Check sheet for the modelled part. Datum: model origin and axes. Units: mm. Face numbers are marked on the shaded views. A direction names the side the tool comes from. Coordinates: 2 decimals unless noted, no trailing zeros. Loops run counter-clockwise (first coordinate to the right, second up) from the corner with the lowest first, then second, coordinate; pieces in that order, holes last. Notation, with made-up numbers: (-14, 45.25) -> (12, 45.25) arc R28 cw to (12, 70.25) -> close; hole circle Ø3 at (85, -10). An arc over 180 degrees is marked (long way). Use one line per item in the form item = value.
from build123d import *

# Parameters (mm, degrees)
F0_W      = 38.7000013143
F0_H      = 33.3000021055
F1_DEPTH  = 25
F3_DEPTH  = 33.3010021055
F4_R      = 50
F5_R      = 0.5
F6_W      = 27.6561714709
F6_H      = 20.6264536828
F7_DEPTH  = 4
F8_W      = 27.6561714709
F8_H      = 16.4114236832
F9_DEPTH  = 10
F10_W     = 27.6561714709
F10_H     = 13.9069892466
F11_DEPTH = 6
F12_W     = 1.1095879599
F12_H     = 33.3000021055
F13_DEPTH = 5


with BuildPart() as f1:
    # F0 (on Top) → F1 (new body)
    with BuildSketch(Plane.XY):
        with Locations((4.9499990419, -5.3999996744)):
            Rectangle(F0_W, F0_H)
    extrude(amount=F1_DEPTH)

    # F2 (on face) → F3 (cut, through all)
    with BuildSketch(Plane.XZ.offset(22.0500007272)):
        Polygon((-14.4000016153, 25), (-14.4000016153, 0), (-3.1048920937, 13.0713665858), (18.2830113918, 19.4805841893), (24.299999699, 25), align=None)
    extrude(amount=-F3_DEPTH, mode=Mode.SUBTRACT)

    # F4
    f4_edges = [f1.edges().sort_by_distance(p)[0] for p in [
        (-3.104892, -5.4, 13.071367),
    ]]
    fillet(f4_edges, radius=F4_R)

    # F5
    f5_edges = [f1.edges().sort_by_distance(p)[0] for p in [
        (24.3, -5.4, 25),
    ]]
    fillet(f5_edges, radius=F5_R)

    # F6 (on face) → F7 (cut)
    with BuildSketch(Plane.YZ.offset(24.299999699)):
        with Locations((-5.37536107, 10.3132268414)):
            Rectangle(F6_W, F6_H)
    extrude(amount=-F7_DEPTH, mode=Mode.SUBTRACT)

    # F8 (on face) → F9 (cut)
    with BuildSketch(Plane.YZ.offset(20.299999699)):
        with Locations((-5.37536107, 8.2057118416)):
            Rectangle(F8_W, F8_H)
    extrude(amount=-F9_DEPTH, mode=Mode.SUBTRACT)

    # F10 (on face) → F11 (cut)
    with BuildSketch(Plane.YZ.offset(10.299999699)):
        with Locations((-5.37536107, 6.9534946233)):
            Rectangle(F10_W, F10_H)
    extrude(amount=-F11_DEPTH, mode=Mode.SUBTRACT)

    # F12 (on face) → F13 (join)
    with BuildSketch(Plane(origin=(0, 0, 0), x_dir=(1, 0, 0), z_dir=(0, 0, -1))):
        with Locations((-13.8452076353, 5.3999996744)):
            Rectangle(F12_W, F12_H)
    extrude(amount=F13_DEPTH)


solid = f1.part
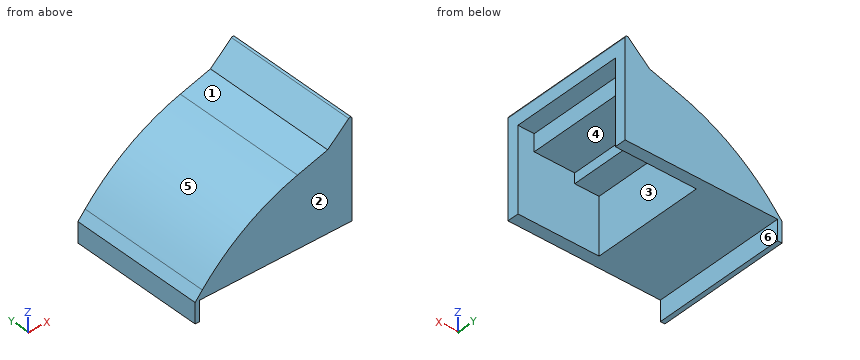
(1) Scan lines: line 1 along Y through (x, z) = (6, 6); line 2 along X through (y, z) = (-18.5, -1.5); line 3 along Z through (x, y) = (2, 8). Record each from-to range of solid material in increasing order.
Established:
line_1 = -22.05 to -19.2, 8.45 to 11.25
line_2 = -14.4 to -13.29
line_3 = 0 to 13.65
(2) Tool access check on the marked faces 4, 5 and 6. Record the directions out of +Z, -Z, +X, -X, +Y, -Y that give a thin tool (end or side, any length) a straight path to the whole face; none if there is none.
Established:
face_4 = -Z, +X
face_5 = +Z, -X, +Y, -Y
face_6 = -Z, +X, +Y, -Y
(3) Section check A-A, the plane y = 0.5. Record the boundary of the cut face in (x, z), plus the area to 3 significant figures.
Established:
outline = (-14.4, -5) -> (-13.29, -5) -> (-13.29, 0) -> (4.3, 0) -> (4.3, 13.91) -> (10.3, 13.91) -> (10.3, 16.41) -> (20.3, 16.41) -> (20.3, 20.63) -> (24.3, 20.63) -> (24.3, 23.86) arc R0.5 ccw to (23.46, 24.23) -> (18.28, 19.48) -> (10.85, 17.25) arc R50 ccw to (-12.63, 2.05) -> (-14.4, 0) -> close
area = 211 mm²
(4) Section check C-C, the plane z = 9.25. Record the boundary of the cut face in (x, y), plus the area to 3 significant figures.
Established:
outline = (-4.94, -22.05) -> (24.3, -22.05) -> (24.3, -19.2) -> (4.3, -19.2) -> (4.3, 8.45) -> (24.3, 8.45) -> (24.3, 11.25) -> (-4.94, 11.25) -> close
area = 421 mm²
(5) Section check D-D, the plane z = -0.5. Record the boundary of the cut face in (x, y).
Established:
outline = (-14.4, -22.05) -> (-13.29, -22.05) -> (-13.29, 11.25) -> (-14.4, 11.25) -> close
(6) Section check B-B, the plane x = 13. Record the boundary of the cut face in (y, z).
Established:
outline = (-22.05, 0) -> (-19.2, 0) -> (-19.2, 16.41) -> (8.45, 16.41) -> (8.45, 0) -> (11.25, 0) -> (11.25, 17.9) -> (-22.05, 17.9) -> close
(7) Go/stop test with flat-tipped pins: P1, Ø3, axis at y = -1, z = 15, coming from the +X side; P2, Ø7, axis at y = -11, z = 4.5, coming from the +X side; P3, Ø4.5, axis at x = 22.5, y = -4, coming from the -Z side. Record where each tip stops, or that it passes through.
Established:
P1 = 20.3
P2 = 4.3
P3 = 16.41
(8) Mould release check, pull along Y, two halves, no side actions. Record for the marked faces 1, 2 and 3: +Y half, -Y half, draft (parallel to the pull), parting line (faces both ways), or undercut.
Established:
face_1 = draft
face_2 = -Y half
face_3 = undercut
